```python
from build123d import *

# Parameters (mm, degrees)
SKETCH1_W           = 12
SKETCH1_H           = 12
SKETCH1_R           = 2.875
BOSS_EXTRUDE1_DEPTH = 5
BOSS_EXTRUDE3_DEPTH = 8
FILLET1_R           = 0.5
SKETCH2_W           = 1.6
SKETCH2_H           = 11.5
CUT_EXTRUDE1_DEPTH  = 6
BOSS_EXTRUDE4_REACH = 14


with BuildPart() as part:
    # Sketch1 → Boss-Extrude1 (new body)
    with BuildSketch(Plane.XY):
        with Locations((2, 0)):
            Rectangle(SKETCH1_W, SKETCH1_H)
        Circle(SKETCH1_R, mode=Mode.SUBTRACT)
    extrude(amount=BOSS_EXTRUDE1_DEPTH)

    # Sketch1_4 → Boss-Extrude3 (add)
    with BuildSketch(Plane.XY):
        with BuildLine():
            ThreePointArc((4.5, 0), (1.060660172, -4.373213921), (-4, -2.061552813))
            Line((-4, -2.061552813), (-4, -6))
            Line((-4, -6), (8, -6))
            Line((8, -6), (8, 6))
            Line((8, 6), (-4, 6))
            Line((-4, 6), (-4, 2.061552813))
            ThreePointArc((-4, 2.061552813), (1.060660172, 4.373213921), (4.5, 0))
        make_face()
    extrude(amount=-BOSS_EXTRUDE3_DEPTH)

    # Fillet1
    fillet1_edges = [part.edges().sort_by_distance(p)[0] for p in [
        (-4, 6, -1.5),
        (8, 6, -1.5),
        (8, -6, -1.5),
        (-4, -6, -1.5),
        (-4, -2.061552813, -4),
        (-4, 2.061552813, -4),
    ]]
    fillet(fillet1_edges, radius=FILLET1_R)

    # Sketch2 → Cut-Extrude1 (cut)
    with BuildSketch(Plane.XZ.offset(6)):
        with Locations((5.7, -2.25)):
            Rectangle(SKETCH2_W, SKETCH2_H)
    extrude(amount=-CUT_EXTRUDE1_DEPTH, mode=Mode.SUBTRACT)

    # Sketch3 → Boss-Extrude4 (add, up to next)
    with BuildSketch(Plane.XZ.offset(6), mode=Mode.PRIVATE) as boss_extrude4_sk1:
        with BuildLine():
            Line((4.9, -8), (5.05, -8))
            ThreePointArc((5.05, -8), (5.65, -7.4), (5.05, -6.8))
            Line((5.05, -6.8), (4.9, -6.8))
            Line((4.9, -6.8), (4.9, -8))
        make_face()
    boss_extrude4_tool1 = extrude(boss_extrude4_sk1.sketch, amount=-BOSS_EXTRUDE4_REACH, mode=Mode.PRIVATE) - part.part
    add(boss_extrude4_tool1.solids().sort_by_distance((5.225053, -6, -7.4))[0])
    # Sketch3 → Boss-Extrude4 (add, up to next)
    with BuildSketch(Plane.XZ.offset(6), mode=Mode.PRIVATE) as boss_extrude4_sk2:
        with BuildLine():
            Line((5.05, -4.8), (4.9, -4.8))
            Line((4.9, -4.8), (4.9, -6))
            Line((4.9, -6), (5.05, -6))
            ThreePointArc((5.05, -6), (5.65, -5.4), (5.05, -4.8))
        make_face()
    boss_extrude4_tool2 = extrude(boss_extrude4_sk2.sketch, amount=-BOSS_EXTRUDE4_REACH, mode=Mode.PRIVATE) - part.part
    add(boss_extrude4_tool2.solids().sort_by_distance((5.225053, -6, -5.4))[0])
    # Sketch3 → Boss-Extrude4 (add, up to next)
    with BuildSketch(Plane.XZ.offset(6), mode=Mode.PRIVATE) as boss_extrude4_sk3:
        with BuildLine():
            Line((5.05, -2.8), (4.9, -2.8))
            Line((4.9, -2.8), (4.9, -4))
            Line((4.9, -4), (5.05, -4))
            ThreePointArc((5.05, -4), (5.65, -3.4), (5.05, -2.8))
        make_face()
    boss_extrude4_tool3 = extrude(boss_extrude4_sk3.sketch, amount=-BOSS_EXTRUDE4_REACH, mode=Mode.PRIVATE) - part.part
    add(boss_extrude4_tool3.solids().sort_by_distance((5.225053, -6, -3.4))[0])
    # Sketch3 → Boss-Extrude4 (add, up to next)
    with BuildSketch(Plane.XZ.offset(6), mode=Mode.PRIVATE) as boss_extrude4_sk4:
        with BuildLine():
            Line((5.05, -0.8), (4.9, -0.8))
            Line((4.9, -0.8), (4.9, -2))
            Line((4.9, -2), (5.05, -2))
            ThreePointArc((5.05, -2), (5.65, -1.4), (5.05, -0.8))
        make_face()
    boss_extrude4_tool4 = extrude(boss_extrude4_sk4.sketch, amount=-BOSS_EXTRUDE4_REACH, mode=Mode.PRIVATE) - part.part
    add(boss_extrude4_tool4.solids().sort_by_distance((5.225053, -6, -1.4))[0])
    # Sketch3 → Boss-Extrude4 (add, up to next)
    with BuildSketch(Plane.XZ.offset(6), mode=Mode.PRIVATE) as boss_extrude4_sk5:
        with BuildLine():
            Line((5.05, 1.2), (4.9, 1.2))
            Line((4.9, 1.2), (4.9, 0))
            Line((4.9, 0), (5.05, 0))
            ThreePointArc((5.05, 0), (5.65, 0.6), (5.05, 1.2))
        make_face()
    boss_extrude4_tool5 = extrude(boss_extrude4_sk5.sketch, amount=-BOSS_EXTRUDE4_REACH, mode=Mode.PRIVATE) - part.part
    add(boss_extrude4_tool5.solids().sort_by_distance((5.225053, -6, 0.6))[0])
    # Sketch3 → Boss-Extrude4 (add, up to next)
    with BuildSketch(Plane.XZ.offset(6), mode=Mode.PRIVATE) as boss_extrude4_sk6:
        with BuildLine():
            Line((5.05, 3.2), (4.9, 3.2))
            Line((4.9, 3.2), (4.9, 2))
            Line((4.9, 2), (5.05, 2))
            ThreePointArc((5.05, 2), (5.65, 2.6), (5.05, 3.2))
        make_face()
    boss_extrude4_tool6 = extrude(boss_extrude4_sk6.sketch, amount=-BOSS_EXTRUDE4_REACH, mode=Mode.PRIVATE) - part.part
    add(boss_extrude4_tool6.solids().sort_by_distance((5.225053, -6, 2.6))[0])


solid = part.part
```
Source: CAD feature listing. Evaluate the final solid. Frame: model axes, mm. A direction names the side the tool comes from. Give positions to 0.01 mm unless a question says otherwise; leave off trailing zeros. Write each loop counter-clockwise with the first axis right and the second up, starting at its lowest first coordinate (ties: lowest second). Pieces come first, ordered by that corner, then holes. Notation, with made-up numbers: (66, 13) - (73, 13) arc R16 ccw to (73, 31) - close; hole circle Ø7 at (15, -30.75). An arc over 180 degrees is marked (long way). One line per item, written item: value. Start each with the question number.
Q1. Section query A-A, the plane x = 0. Return the cut outline in (y, z) (3 decimals).
Q2. Material intervals for probe 1 along Y at (x, z) = (0, 1.4) (3 decimals); probe 2 along Z at (x, y) = (2.25, -3); probe 3 along X at (y, z) = (-0.25, 1.5), sorted ascending. Write a range as from..to.
Q3. Set-up query: faces 5 (the face through (3.2, 0.1, 5)), 6 (the face through (6.5, -3, -2)), 7 (the face through (-3.69, -3.11, -4.06)), 8 (the face through (6, -3, 3.5)). Return all of +Z, -Z, +X, -X, +Y, -Y with unobstructed straight access to the full face (end or side cutting, diameter ignored); none if empty.
Q4. First-contact query: pin 1 Ø6.5 at (x, y) = (0, 0) entering from -Z; pin 2 Ø0.5 at (x, y) = (6, -4) entering from -Z. Flat tips, straight axial feed; report the tip coordinate or a pass-through.
Q5. Section query B-B, the plane z = 0.6. Return the cut outline in (x, y) (3 decimals), then the cut area to 3 significant figures.
Q6. Section query C-C, the plane y = 2. Return the cut outline in (x, z), then the cut area to 3 significant figures.
Q7. Draft query along X for faces 1 (the face through (-4, 0, 1)), 2 (the face through (5.65, -3.04, -3.41)), 3 (the face through (8, 0, -1)), 4 (the face through (2, 6, -1)). Return one class per face: +X half, -X half, draft (parallel to the pull), parting line (faces both ways), or undercut.
Answer:
1. outline: (-6, -8) - (-4.5, -8) - (-4.5, 0) - (-2.875, 0) - (-2.875, 5) - (-6, 5) - close; (2.875, 0) - (4.5, 0) - (4.5, -8) - (6, -8) - (6, 5) - (2.875, 5) - close
2. probe 1: y = -6..-2.875, 2.875..6
2. probe 2: z = 0..5
2. probe 3: x = -4..-2.86, 2.86..4.9, 6.5..8
3. face 5: +Z, +X, -X, +Y, -Y
3. face 6: -Z, -Y
3. face 7: -Z
3. face 8: -Y
4. pin 1: stops at z = 0
4. pin 2: stops at z = 3.5
5. outline: (-4, -5.5) arc R0.5 ccw to (-3.5, -6) - (5.65, -6) - (5.65, 0) - (6.5, 0) - (6.5, -6) - (7.5, -6) arc R0.5 ccw to (8, -5.5) - (8, 5.5) arc R0.5 ccw to (7.5, 6) - (-3.5, 6) arc R0.5 ccw to (-4, 5.5) - close; hole circle Ø5.75 at (0, 0)
5. area: 113 mm2
6. outline: (-4, 0) - (-2.07, 0) - (-2.07, 5) - (-4, 5) - close; (2.07, 0) - (4.03, 0) - (4.03, -8) - (8, -8) - (8, 5) - (2.07, 5) - close
6. area: 71.1 mm2
7. face 1: -X half
7. face 2: undercut
7. face 3: +X half
7. face 4: draft
